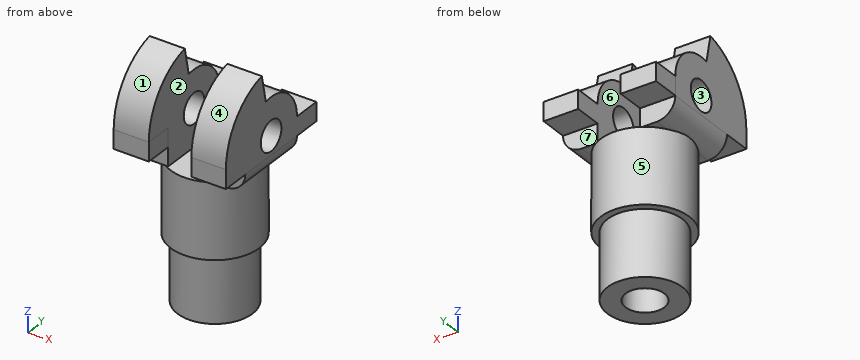
Autodesk Inventor part; units mm, degrees
ref_plane "YZ Plane" through (0, 0, 0) normal (1, 0, 0) x (0, 1, 0)
ref_plane "XZ Plane" through (0, 0, 0) normal (0, 1, 0) x (-1, 0, 0)
ref_plane "XY Plane" through (0, 0, 0) normal (0, 0, 1) x (1, 0, 0)
sketch "Sketch1" plane through (0, 0, 0) normal (0, 0, 1) x (1, 0, 0)
  circle A0 centre (0, 0) radius 2
  circle A1 centre (0, 0) radius 4
  dimension "d0" = 4
  dimension "d1" = 8
extrude "Extrusion1" add sketch "Sketch1" along normal blind 15
sketch "Sketch2" plane through (0, 0, 15) normal (0, 0, 1) x (1, 0, 0)
  circle A0 centre (0, 0) radius 4
  line L0 (0, 4) -> (6, 4)
  line L1 (6, 4) -> (6, -4)
  line L2 (6, -4) -> (0, -4)
  line L3 (0, -4) -> (0, 4)
  line L4 (0, 4) -> (-6, 4)
  line L5 (-6, 4) -> (-6, -4)
  line L6 (-6, -4) -> (0, -4)
  line L7 (0, -4) -> (0, 4)
  dimension "d4" = 6
  dimension "d5" = 6
extrude "Extrusion2" add sketch "Sketch2" along normal blind 8
sketch "Sketch3" plane through (0, 0, 23) normal (0, 0, 1) x (1, 0, 0)
  line L0 (6, 4) -> (-6, 4)
  line L1 (-6, -4) -> (6, -4)
  line L2 (-2.2377, 4) -> (2.306, 4)
  line L3 (2.306, 4) -> (2.306, -4)
  line L4 (2.306, -4) -> (-2.2377, -4)
  line L5 (-2.2377, -4) -> (-2.2377, 4)
  point P0 (0, 0)
extrude "Extrusion3" cut sketch "Sketch3" against normal blind 8
sketch "Sketch4" plane through (0, 0, 15) normal (0, 0, -1) x (-1, 0, 0)
  circle A0 centre (0, 0) radius 4
  circle A1 centre (0, 0) radius 4.731
extrude "Extrusion4" add sketch "Sketch4" along normal blind 8
sketch "Sketch5" plane through (6, -4, 15) normal (1, 0, 0) x (0, 0, -1)
  line L0 (0, 8) -> (-8, 8)
  line L1 (0, 0) -> (-8, 0)
  line L2 (-8, 8) -> (0, 8)
  line L3 (0, 8) -> (0, 0)
  line L4 (0, 0) -> (-8, 0)
  line L5 (-8, 0) -> (-8, 8)
  circle A0 centre (-4, 4) radius 1.6
  circle A1 centre (-4, 4) radius 4
  point P0 (15, 4)
  point P1 (-8, 4)
  point P2 (-4, 8)
  point P3 (-4, 0)
  dimension "d12" = 3.2
extrude "Extrusion5" cut sketch "Sketch5" against normal blind 14 contours A1 L5 L0 | A1 L1 L5 | A0
fillet "Fillet1" radius 2 2 edges at (-6, 0, 15) (6, 0, 15)
sketch "Sketch7" plane through (2.306, 4, 15) normal (0, 1, 0) x (1, 0, 0)
  point P0 (-2.306, 15)
sketch "Sketch8" plane through (2.306, 4, 15) normal (0, 1, 0) x (1, 0, 0)
  line L0 (0, -4) -> (3.694, -4)
  line L1 (0, 0) -> (0, -4)
  line L2 (3.694, -4) -> (0, -4)
  line L3 (0, -4) -> (0, -2)
  line L4 (0, -2) -> (3.694, -2)
  line L5 (3.694, -2) -> (3.694, -4)
  line L6 (-4.5455, -4) -> (-8.3301, -4)
  line L7 (-8.3301, -4) -> (-8.3301, -2)
  line L8 (-8.3301, -2) -> (-4.5455, -2)
  line L9 (-4.5455, -2) -> (-4.5455, -4)
  point P0 (-2.306, 15)
extrude "Extrusion7" add sketch "Sketch8" along normal blind 3
sketch "Sketch9" plane through (-2.5263, -4, 15) normal (0, -1, 0) x (1, 0, 0)
  line L0 (-3.4737, 2) -> (-3.4737, 4)
  line L1 (0.2868, 2) -> (-3.4978, 2)
  line L2 (-3.4737, 4) -> (0.2868, 4)
  line L3 (0.2868, 4) -> (0.2868, 2)
  line L4 (0.2868, 2) -> (-3.4737, 2)
  line L5 (-3.4737, 2) -> (-3.4737, 4)
  line L6 (4.8006, 4) -> (8.5263, 4)
  line L7 (8.5263, 4) -> (8.5263, 2)
  line L8 (8.5263, 2) -> (4.8006, 2)
  line L9 (4.8006, 2) -> (4.8006, 4)
  point P0 (2.5263, -15)
extrude "Extrusion8" add sketch "Sketch9" along normal blind 3
sketch "Sketch10" plane through (6, 4, 17) normal (1, 0, 0) x (0, 0, -1)
  circle A0 centre (-1.9999, -4) radius 7
  circle A1 centre (-2, -4) radius 1.6
  circle A2 centre (-2, -4) radius 4
  line L0 (-2, -8) -> (-1.9999, -11)
  line L1 (-2, -4) -> (-8.8503, -5.4392)
  point P0 (17, -4)
  point P1 (-5.9145, -4.8224)
  dimension "d24" = 14
extrude "Extrusion9" add sketch "Sketch10" against normal blind 12 contours L1 A2 L0 A0 picked at (-2.5257, -9.94)
sketch "Sketch11" plane through (-2.5263, -4, 15) normal (0, -1, 0) x (1, 0, 0)
  line L0 (0, 0) -> (0.2886, 0)
  line L1 (0.2886, 0) -> (4.8323, 0)
  line L2 (4.8323, 0) -> (4.8323, 13.1536)
  line L3 (4.8323, 13.1536) -> (0.2886, 13.1536)
  line L4 (0.2886, 13.1536) -> (0.2886, 0)
  point P0 (2.5263, -15)
extrude "Extrusion10" cut sketch "Sketch11" along normal mid plane 12
sketch "Sketch12" plane through (0, 0, 0) normal (0, 0, -1) x (-1, 0, 0)
  circle A0 centre (0, 0) radius 2.075
  dimension "d29" = 4.15
extrude "Extrusion11" cut sketch "Sketch12" against normal blind 20
sketch "Sketch13" plane through (0, 0, 15) normal (0, 0, 1) x (1, 0, 0)
  circle A0 centre (0, 0) radius 2.2168
extrude "Extrusion12" add sketch "Sketch13" against normal blind 1
properties part number "hingejoint2"
CAD build for the part. Positions are in the model's coordinates, mm. Face numbers are marked on the shaded views. A direction names the side the tool comes from. Round coordinates to 2 decimals unless told otherwise and drop trailing zeros. Write each loop counter-clockwise with the first axis right and the second up, starting at its lowest first coordinate (ties: lowest second). Pieces come first, ordered by that corner, then holes. Notation, with made-up numbers: M -14.5,76 L 21.5,76 A24 ccw 21.5,96 Z; hole C 30.5,80.5 d4. An arc over 180 degrees is marked long. Use a Markdown table: item, result. Add a question column.
1. Pull direction Z, two halves, no side cores. Call the marked faces 1, 2 and 3: released by +Z, released by -Z, zero draft, split by the parting line, or undercut.
2. 3-axis set-ups, long thin cutter, end or side, ignore diameter. For the marked faces 4, 5, 6 and 7: which of +Z, -Z, +X, -X, +Y, -Y reach the whole face in a straight line?
3. Drill centre lines: probe 1 along X at (y, z) = (-1, 22.5); probe 2 along Z at (x, y) = (5, 5.75); probe 3 along Z at (x, y) = (4.25, -0.75). Where is each one in solid material? Low to high.
4. Slice it at D-D on x = -3.5. Give the cut face in (y, z), then the cut area to 3 significant figures.
5. Slice it at A-A on y = 0. Give the cut face in (x, z) (3 decimals), then the cut area to 3 significant figures.
6. Slice it at B-B on z = 21.75. Give the cut face in (x, y), then the cut area to 3 significant figures.
7. Flat gauge pins, fed straight in: P1, Ø3, axis at y = 0, z = 7.5, coming from the +X side; P2, Ø1, axis at x = 5, z = 16, coming from the -Y side; P3, Ø6, axis at x = 0.5, z = 4.5, coming from the -Y side. Where does each tip first touch, or does it go through?
Reply:
| question | item | result |
|---|---|---|
| 1 | face 1 | released by +Z |
| 1 | face 2 | zero draft |
| 1 | face 3 | undercut |
| 2 | face 4 | +Z, +X, -X, -Y |
| 2 | face 5 | -Z |
| 2 | face 6 | +Z, +Y, -Y |
| 2 | face 7 | +X, -X, +Y |
| 3 | probe 1 | x = -6 to -2.24, 2.31 to 6 |
| 3 | probe 2 | z = 17 to 19 |
| 3 | probe 3 | z = 7 to 17.59, 20.41 to 22.93 |
| 4 | outline | M -7,17 L -4,17 L -4,15 L -3.18,15 L -3.18,7 L -1.94,7 L -1.94,0 L 1.94,0 L 1.94,7 L 3.18,7 L 3.18,15 L 4,15 L 4,17 L 7,17 L 7,19 L 4,19 A4 ccw -0.82,22.91 L -1.44,25.85 A7 ccw -7,19 Z; hole C 0,19 d3.2 |
| 4 | area | 162 mm^2 |
| 5 | outline | M -6,17 A2 ccw -4.731,15.138 L -4.731,7 L -4,7 L -4,0 L -2.075,0 L -2.075,14 L 2.075,14 L 2.075,0 L 4,0 L 4,7 L 4.731,7 L 4.731,15.138 A2 ccw 6,17 L 6,17.4 L 2.306,17.4 L 2.306,15 L -2.238,15 L -2.238,17.4 L -6,17.4 Z; M -6,20.6 L -2.238,20.6 L -2.238,23 L -6,23 Z; M 2.306,20.6 L 6,20.6 L 6,23 L 2.306,23 Z |
| 5 | area | 108 mm^2 |
| 6 | outline | M -6,-6.44 L -2.24,-6.44 L -2.24,2.9 L -6,2.9 Z; M 2.31,-6.44 L 6,-6.44 L 6,2.9 L 2.31,2.9 Z |
| 6 | area | 69.7 mm^2 |
| 7 | P1 | stops at x = 4.73 |
| 7 | P2 | stops at y = -4 |
| 7 | P3 | stops at y = -4.73 |
